from build123d import *

# Parameters (mm, degrees)
CHAMFER1_SIZE = 1.27


with BuildPart() as part:
    # Sketch2 → Revolve1 (revolve)
    with BuildSketch(Plane(origin=(0, 0, 0), x_dir=(0, 0, -1), z_dir=(1, 0, 0)), mode=Mode.PRIVATE) as revolve1_sk:
        Polygon((0, 38.1), (-15.875, 38.1), (-15.875, 30.465422705), (-9.525, 29.345746377), (-9.525, 21.711169082), (-9.525, 14.076591787), (-19.05, 12.397077295), (-19.05, 4.7625), (0, 4.7625), align=None)
    revolve(revolve1_sk.sketch.rotate(Axis((0, 0, 19.05), (0, 0, -1)), 180), axis=Axis((0, 0, 19.05), (0, 0, -1)))

    # Chamfer1
    chamfer1_edges = [part.edges().sort_by_distance(p)[0] for p in [
        (0, 38.1, 15.875),
    ]]
    chamfer(chamfer1_edges, length=CHAMFER1_SIZE)

    # Mirror2: part across plane


with BuildPart() as part_1:
    add(part.part)
    add(part.part.mirror(Plane.XY))


solid = part_1.part
Work out the finished part from the listing and answer in its coordinate system (mm). Give positions to 0.01 mm unless a question says otherwise; leave off trailing zeros. Write each loop counter-clockwise with the first axis right and the second up, starting at its lowest first coordinate (ties: lowest second). Pieces come first, ordered by that corner, then holes.
Q1. The part is cut by section D-D on z = -11.5. Give the vertices of the cut face in (x, y) (1 decimal), and give its area (3 significant figures).
Answer:
outline: circle Ø76.2 at (0, 0); circle Ø27.5 at (0, 0); hole circle Ø59.4 at (0, 0); hole circle Ø9.5 at (0, 0)
area: 2,310 mm2
Q2. For a pull along X with two mould halves and no side action, classify faces 1 (the face through (-27.5, 13.8, -15.875)), 2 (the face through (-7, -13, 9.525)), 3 (the face through (-7, -13, -9.525)) as released by +X, released by -X, zero draft, split by the parting line, or undercut.
Answer:
face 1: zero draft
face 2: undercut
face 3: undercut
Q3. Straight lines are drawn through the part: L1, parallel to X at y = 0, z = 11; L2, parallel to Y at x = 7.5, z = 15.5; L3, parallel to X at y = -11, z = 12.5. For each, find the intervals that lie inside material, in ascending order.
Answer:
L1: x = -38.1 to -29.61, -13.82 to -4.76, 4.76 to 13.82, 29.61 to 38.1
L2: y = -36.44 to -29.46, -10.65 to 10.65, 29.46 to 36.44
L3: x = -36.48 to -27.77, -7.92 to 7.92, 27.77 to 36.48
Q4. The part is cut by section C-C on z = 3. Give the vertices of the cut face in (x, y) (1 decimal).
Answer:
outline: circle Ø76.2 at (0, 0); hole circle Ø9.5 at (0, 0)
Q5. Given pin 1 (1.5 mm diameter, centred on y = -7.5, z = 6.5, fed in from -X); pin 2 (12 mm diameter, centred on x = 23, z = 14, fed in from -Y); pin 3 (10 mm diameter, centred on x = -17, y = 16, fed in from -Z) (3 decimals), each flat-ended and moving along its own axis, determine where each tip first touches the part or whether it passes through.
Answer:
pin 1: stops at x = -37.5
pin 2: stops at y = -34.1
pin 3: stops at z = -9.525
